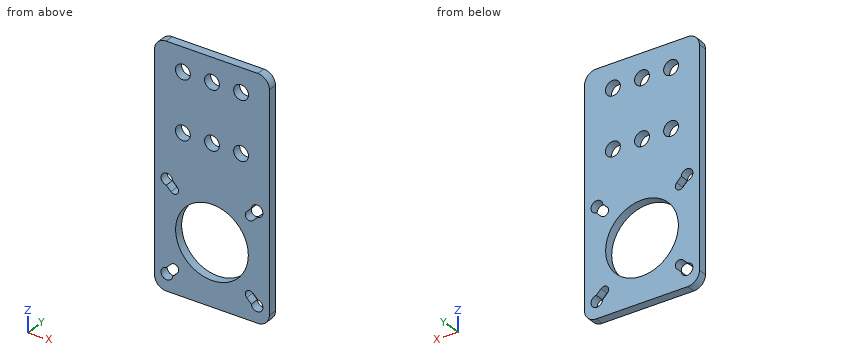
```python
from build123d import *

# Parameters (mm, degrees)
SKETCH1_R           = 12.5
SKETCH1_R_2         = 2.55
BOSS_EXTRUDE1_DEPTH = 3
SKETCH2_R           = 2
CUT_EXTRUDE1_DEPTH  = 10


with BuildPart() as part:
    # Sketch1 → Boss-Extrude1 (new body)
    with BuildSketch(Plane(origin=(0, 0, 0), x_dir=(1, 0, 0), z_dir=(0, 1, 0))):
        with BuildLine():
            Line((15.75, -60.75), (-15.75, -60.75))
            ThreePointArc((-15.75, -60.75), (-18.578427125, -59.578427125), (-19.75, -56.75))
            Line((-19.75, -56.75), (-19.75, 17.25))
            ThreePointArc((-19.75, 17.25), (-18.578427125, 20.078427125), (-15.75, 21.25))
            Line((-15.75, 21.25), (15.75, 21.25))
            ThreePointArc((15.75, 21.25), (18.578427125, 20.078427125), (19.75, 17.25))
            Line((19.75, 17.25), (19.75, -56.75))
            ThreePointArc((19.75, -56.75), (18.578427125, -59.578427125), (15.75, -60.75))
        make_face()
        Circle(SKETCH1_R, mode=Mode.SUBTRACT)
        with Locations((10, -52.55)):
            Circle(SKETCH1_R_2, mode=Mode.SUBTRACT)
        with Locations((10, -32.55)):
            Circle(SKETCH1_R_2, mode=Mode.SUBTRACT)
        with Locations((0, -52.55)):
            Circle(SKETCH1_R_2, mode=Mode.SUBTRACT)
        with Locations((0, -32.55)):
            Circle(SKETCH1_R_2, mode=Mode.SUBTRACT)
        with Locations((-10, -52.55)):
            Circle(SKETCH1_R_2, mode=Mode.SUBTRACT)
        with Locations((-10, -32.55)):
            Circle(SKETCH1_R_2, mode=Mode.SUBTRACT)
        with BuildLine():
            Line((11.903984489, 14.096015511), (14.403984489, 16.596015511))
            ThreePointArc((14.403984489, 16.596015511), (16.596015511, 16.596015511), (16.596015511, 14.403984489))
            Line((16.596015511, 14.403984489), (14.096015511, 11.903984489))
            ThreePointArc((14.096015511, 11.903984489), (11.903984489, 11.903984489), (11.903984489, 14.096015511))
        make_face(mode=Mode.SUBTRACT)
        with BuildLine():
            Line((-11.903984489, 14.096015511), (-14.403984489, 16.596015511))
            ThreePointArc((-14.403984489, 16.596015511), (-16.596015511, 16.596015511), (-16.596015511, 14.403984489))
            Line((-16.596015511, 14.403984489), (-14.096015511, 11.903984489))
            ThreePointArc((-14.096015511, 11.903984489), (-11.903984489, 11.903984489), (-11.903984489, 14.096015511))
        make_face(mode=Mode.SUBTRACT)
        with BuildLine():
            Line((-11.903984489, -14.096015511), (-14.403984489, -16.596015511))
            ThreePointArc((-14.403984489, -16.596015511), (-16.596015511, -16.596015511), (-16.596015511, -14.403984489))
            Line((-16.596015511, -14.403984489), (-14.096015511, -11.903984489))
            ThreePointArc((-14.096015511, -11.903984489), (-11.903984489, -11.903984489), (-11.903984489, -14.096015511))
        make_face(mode=Mode.SUBTRACT)
        with BuildLine():
            Line((11.903984489, -14.096015511), (14.403984489, -16.596015511))
            ThreePointArc((14.403984489, -16.596015511), (16.596015511, -16.596015511), (16.596015511, -14.403984489))
            Line((16.596015511, -14.403984489), (14.096015511, -11.903984489))
            ThreePointArc((14.096015511, -11.903984489), (11.903984489, -11.903984489), (11.903984489, -14.096015511))
        make_face(mode=Mode.SUBTRACT)
    extrude(amount=BOSS_EXTRUDE1_DEPTH)

    # Sketch2 → Cut-Extrude1 (cut)
    with BuildSketch(Plane(origin=(0, 3, 0), x_dir=(1, 0, 0), z_dir=(0, 1, 0))):
        with Locations((-15.5, 15.5)):
            Circle(SKETCH2_R)
        with Locations((15.5, 15.5)):
            Circle(SKETCH2_R)
        with Locations((-15.5, -15.5)):
            Circle(SKETCH2_R)
        with Locations((15.5, -15.5)):
            Circle(SKETCH2_R)
    extrude(amount=-CUT_EXTRUDE1_DEPTH, mode=Mode.SUBTRACT)


solid = part.part
```
Can you work these out from the model? Positions are in its coordinate system, mm. Coordinates: 2 decimals unless noted, no trailing zeros. Loops run counter-clockwise (first coordinate to the right, second up) from the corner with the lowest first, then second, coordinate; pieces in that order, holes last. Notation, with made-up numbers: (-26.75, -6) -> (-4.75, -6) arc R24 cw to (-4.75, 18) -> close; hole circle Ø5 at (-16.75, 13). An arc over 180 degrees is marked (long way). Answer as a JSON object with one key per item and string values.
1) If I drill on line 1 (X direction, y = 1.9, z = 32.55); line 2 (Z direction, x = 0, y = 1.2); line 3 (Z direction, x = -15.5, y = 1.3), over which ranges is the centre line in solid material (lowest first)?
Results:
{"line 1": "x = -19.75 to -12.55, -7.45 to -2.55, 2.55 to 7.45, 12.55 to 19.75", "line 2": "z = -21.25 to -12.5, 12.5 to 30, 35.1 to 50, 55.1 to 60.75", "line 3": "z = -21.25 to -17.5, -13.31 to 13.31, 17.5 to 60.75"}
2) Imagine slicing it at C-C (y = 2.2). Count the separate pieces of the cut face and the enclosed holes in it, then the cut area to 3 significant figures.
Results:
{"separate pieces": "1", "enclosed holes": "11", "area": "2,520 mm^2"}
3) Imagine slicing it at A-A (x = 10). Please give me the cut outline in (y, z), then the cut area to 3 significant figures.
Results:
{"outline": "(0, -21.25) -> (3, -21.25) -> (3, -7.5) -> (0, -7.5) -> close; (0, 7.5) -> (3, 7.5) -> (3, 30) -> (0, 30) -> close; (0, 35.1) -> (3, 35.1) -> (3, 50) -> (0, 50) -> close; (0, 55.1) -> (3, 55.1) -> (3, 60.75) -> (0, 60.75) -> close", "area": "170 mm^2"}
4) Imagine slicing it at B-B (z = -5). Please give me the cut outline in (x, y), then the cut area to 3 significant figures.
Results:
{"outline": "(-19.75, 0) -> (-11.46, 0) -> (-11.46, 3) -> (-19.75, 3) -> close; (11.46, 0) -> (19.75, 0) -> (19.75, 3) -> (11.46, 3) -> close", "area": "49.8 mm^2"}
5) Imagine slicing it at D-D (x = -5.5). Please give me the cut outline in (y, z).
Results:
{"outline": "(0, -21.25) -> (3, -21.25) -> (3, -11.22) -> (0, -11.22) -> close; (0, 11.22) -> (3, 11.22) -> (3, 60.75) -> (0, 60.75) -> close"}
